Here's how the part is built. I have some questions about the finished solid (model axes, mm). Face numbers are marked on the shaded views. A direction names the side the tool comes from. Round coordinates to 2 decimals unless told otherwise and drop trailing zeros. Loops run counter-clockwise (first coordinate to the right, second up) from the corner with the lowest first, then second, coordinate; pieces in that order, holes last. Notation, with made-up numbers: M -40,72 L 2,72 A31 ccw 2,103 Z; hole C -20,58.25 d3. An arc over 180 degrees is marked long. Answer as a JSON object with one key per item and string values.
from build123d import *

# Parameters (mm, degrees)
CYLINDER067_R     = 0.25
CYLINDER067_DEPTH = 10
CYLINDER068_R     = 0.25
CYLINDER068_DEPTH = 10
CYLINDER069_R     = 0.25
CYLINDER069_DEPTH = 10
CYLINDER070_R     = 0.25
CYLINDER070_DEPTH = 10
CYLINDER066_R     = 0.25
CYLINDER066_DEPTH = 10
BOX094_W          = 13
BOX094_H          = 4
BOX094_DEPTH      = 1.4
CYLINDER065_R     = 3.5
CYLINDER065_DEPTH = 4
FILLET027_R       = 2
FILLET030_R       = 1
FILLET031_R       = 1
CYLINDER064_R     = 1.65
CYLINDER064_DEPTH = 10
CYLINDER063_R     = 1.65
CYLINDER063_DEPTH = 10
BOX093_W          = 33.5
BOX093_H          = 14
BOX093_DEPTH      = 3
CYLINDER062_R     = 2
CYLINDER062_DEPTH = 3
CYLINDER061_R     = 7
CYLINDER061_DEPTH = 3
BOX092_W          = 24
BOX092_H          = 14
BOX092_DEPTH      = 23


with BuildPart() as cilindro067:
    # Cylinder067 → Cylinder067 (new body)
    with BuildSketch(Plane(origin=(19, 7, 25), x_dir=(1, 0, 0), z_dir=(0, 0, 1))):
        Circle(CYLINDER067_R)
    extrude(amount=CYLINDER067_DEPTH)


with BuildPart() as cilindro068:
    # Cylinder068 → Cylinder068 (new body)
    with BuildSketch(Plane(origin=(17, 7, 25), x_dir=(1, 0, 0), z_dir=(0, 0, 1))):
        Circle(CYLINDER068_R)
    extrude(amount=CYLINDER068_DEPTH)


with BuildPart() as cilindro069:
    # Cylinder069 → Cylinder069 (new body)
    with BuildSketch(Plane(origin=(15, 7, 27), x_dir=(1, 0, 0), z_dir=(0, 0, 1))):
        Circle(CYLINDER069_R)
    extrude(amount=CYLINDER069_DEPTH)


with BuildPart() as cilindro070:
    # Cylinder070 → Cylinder070 (new body)
    with BuildSketch(Plane(origin=(13, 7, 27), x_dir=(1, 0, 0), z_dir=(0, 0, 1))):
        Circle(CYLINDER070_R)
    extrude(amount=CYLINDER070_DEPTH)


with BuildPart() as cilindro066:
    # Cylinder066 → Cylinder066 (new body)
    with BuildSketch(Plane(origin=(21, 7, 25), x_dir=(1, 0, 0), z_dir=(0, 0, 1))):
        Circle(CYLINDER066_R)
    extrude(amount=CYLINDER066_DEPTH)


with BuildPart() as cubo094:
    # Box094 → Box094 (new body)
    with BuildSketch(Plane(origin=(9.8, 5, 28.6), x_dir=(1, 0, 0), z_dir=(0, 0, 1))):
        with Locations((6.5, 2)):
            Rectangle(BOX094_W, BOX094_H)
    extrude(amount=BOX094_DEPTH)


with BuildPart() as fillet031:
    # Cylinder065 → Cylinder065 (new body)
    with BuildSketch(Plane(origin=(7, 7, 26), x_dir=(1, 0, 0), z_dir=(0, 0, 1))):
        Circle(CYLINDER065_R)
    extrude(amount=CYLINDER065_DEPTH)

    # Fusion067: union Cubo094
    add(cubo094.part)

    # Fillet027
    fillet027_edges = [fillet031.edges().sort_by_distance(p)[0] for p in [
        (9.872281, 5, 29.3),
    ]]
    fillet(fillet027_edges, radius=FILLET027_R)

    # Fillet030
    fillet030_edges = [fillet031.edges().sort_by_distance(p)[0] for p in [
        (22.8, 5, 29.3),
    ]]
    fillet(fillet030_edges, radius=FILLET030_R)

    # Fillet031
    fillet031_edges = [fillet031.edges().sort_by_distance(p)[0] for p in [
        (22.8, 9, 29.3),
    ]]
    fillet(fillet031_edges, radius=FILLET031_R)


with BuildPart() as cilindro064:
    # Cylinder064 → Cylinder064 (new body)
    with BuildSketch(Plane(origin=(26.8, 7, 12), x_dir=(1, 0, 0), z_dir=(0, 0, 1))):
        Circle(CYLINDER064_R)
    extrude(amount=CYLINDER064_DEPTH)


with BuildPart() as cilindro063:
    # Cylinder063 → Cylinder063 (new body)
    with BuildSketch(Plane(origin=(-3.2, 7, 12), x_dir=(1, 0, 0), z_dir=(0, 0, 1))):
        Circle(CYLINDER063_R)
    extrude(amount=CYLINDER063_DEPTH)


with BuildPart() as cubo093:
    # Box093 → Box093 (new body)
    with BuildSketch(Plane(origin=(-5, 0, 16), x_dir=(1, 0, 0), z_dir=(0, 0, 1))):
        with Locations((16.75, 7)):
            Rectangle(BOX093_W, BOX093_H)
    extrude(amount=BOX093_DEPTH)


with BuildPart() as cilindro062:
    # Cylinder062 → Cylinder062 (new body)
    with BuildSketch(Plane(origin=(14, 7, 23), x_dir=(1, 0, 0), z_dir=(0, 0, 1))):
        Circle(CYLINDER062_R)
    extrude(amount=CYLINDER062_DEPTH)


with BuildPart() as fusion064:
    # Cylinder061 → Cylinder061 (new body)
    with BuildSketch(Plane(origin=(7, 7, 23), x_dir=(1, 0, 0), z_dir=(0, 0, 1))):
        Circle(CYLINDER061_R)
    extrude(amount=CYLINDER061_DEPTH)

    # Fusion064: union Cilindro062
    add(cilindro062.part)


with BuildPart() as servo006:
    # Box092 → Box092 (new body)
    with BuildSketch(Plane.XY):
        with Locations((12, 7)):
            Rectangle(BOX092_W, BOX092_H)
    extrude(amount=BOX092_DEPTH)

    # Fusion065: union Fusion064
    add(fusion064.part)

    # Fusion066: union Cubo093
    add(cubo093.part)

    # Cut086: cut Cilindro063
    add(cilindro063.part, mode=Mode.SUBTRACT)

    # Cut087: cut Cilindro064
    add(cilindro064.part, mode=Mode.SUBTRACT)

    # Fusion068: union Fillet031
    add(fillet031.part)

    # Cut088: cut Cilindro066
    add(cilindro066.part, mode=Mode.SUBTRACT)

    # Cut089: cut Cilindro070
    add(cilindro070.part, mode=Mode.SUBTRACT)

    # Cut090: cut Cilindro069
    add(cilindro069.part, mode=Mode.SUBTRACT)

    # Cut091: cut Cilindro068
    add(cilindro068.part, mode=Mode.SUBTRACT)

    # Cut092: cut Cilindro067
    add(cilindro067.part, mode=Mode.SUBTRACT)


with BuildPart() as servo006_1:
    # Cut092 placement: moved
    add(servo006.part.moved(Location((-12, 27, -6))))


solid = servo006_1.part
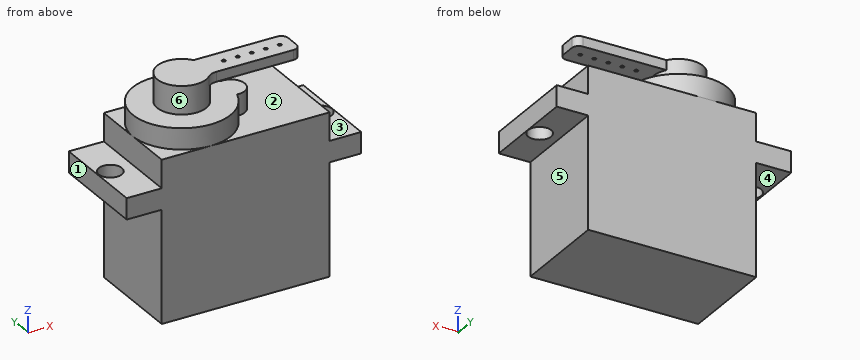
Item 1: I want a section at D-D on x = 14.8. List the corners of the cut face in (y, z) for me.
Solution:
{"outline": "M 27,10 L 32.35,10 L 32.35,13 L 27,13 Z; M 35.65,10 L 41,10 L 41,13 L 35.65,13 Z"}
Item 2: For the marked faces 4, 5 and 6, which set-ups out of +Z, -Z, +X, -X, +Y, -Y let a thin tool reach every point of the face, with its end or its side?
Solution:
{"face 4": "-Z, -X, +Y, -Y", "face 5": "-Z, +X, +Y, -Y", "face 6": "none"}
Item 3: I want a section at B-B on z = 12.25. List the corners of the cut face in (x, y) for me.
Solution:
{"outline": "M -17,27 L 16.5,27 L 16.5,41 L -17,41 Z; hole C -15.2,34 d3.3; hole C 14.8,34 d3.3"}
Item 4: For P1, Ø5.5, axis at x = -13.5, y = 37.5, coming from the +Z side; P2, Ø2, axis at y = 34.5, z = 15.5, coming from the -X side; P3, Ø2, axis at y = 36.5, z = 15, coming from the +X side; P4, Ø2.5, axis at x = 14.8, y = 34, coming from the -Z side, each with a flat end and sliding along its axis, tell me the tip position at first contact or that it passes through.
Solution:
{"P1": "stops at z = 20", "P2": "stops at x = -12", "P3": "stops at x = 12", "P4": "passes through"}
Item 5: If I drill on L1, parallel to X at y = 34, z = 23.1; L2, parallel to Y at x = 14.8, z = 12.3; L3, parallel to Y at x = 1, z = 23.6, over which ranges is the centre line in solid material (lowest first)? Write a range as from..to.
Solution:
{"L1": "x = -8.5..0.75, 1.25..2.75, 3.25..4.75, 5.25..6.75, 7.25..8.75, 9.25..10.8", "L2": "y = 27..32.35, 35.65..41", "L3": "y = 32..33.75, 34.25..36"}
Item 6: I want a section at A-A on x = 6. List the corners of the cut face in (y, z) for me.
Solution:
{"outline": "M 27,-6 L 41,-6 L 41,17 L 27,17 Z; M 32,22.6 L 36,22.6 L 36,24 L 32,24 Z"}
Item 7: We'd pull the mould along Z, two halves only. Please class the marked faces 1, 2 and 3: +Z half, -Z half, draft (parallel to the pull), parting line (faces both ways), or undercut.
Solution:
{"face 1": "draft", "face 2": "undercut", "face 3": "+Z half"}
Item 8: I want a section at C-C on y = 30. List the corners of the cut face in (x, z) for me.
Solution:
{"outline": "M -17,10 L -12,10 L -12,-6 L 12,-6 L 12,10 L 16.5,10 L 16.5,13 L 12,13 L 12,17 L 0.74,17 L 0.74,20 L -10.74,20 L -10.74,17 L -12,17 L -12,13 L -17,13 Z"}
